Geometry: final body of the model. Coordinates: model frame, mm. Face numbers are marked on the shaded views. A direction names the side the tool comes from. Give positions to 0.01 mm unless a question says otherwise; leave off trailing zeros. Loops run counter-clockwise (first coordinate to the right, second up) from the corner with the lowest first, then second, coordinate; pieces in that order, holes last.
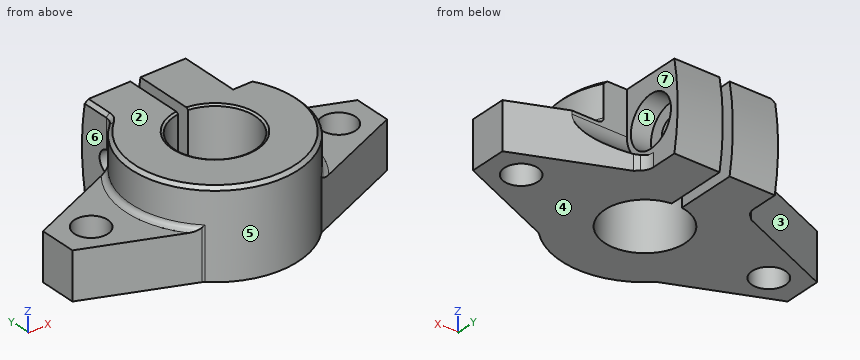
from build123d import *

# Parameters (mm, degrees)
BOSS_EXTRUDE1_DEPTH                                 = 13
CUT_EXTRUDE1_DEPTH                                  = 24.780243901
CUT_EXTRUDE1_DEPTH_BACK                             = 24.780243901
FILLET1_R                                           = 2
BOSS_EXTRUDE2_DEPTH                                 = 7
HOLE_WIZARD_5_0_5_1_D                               = 5
HOLE_WIZARD_5_0_5_1_DEPTH                           = 10
HOLE_WIZARD_5_0_5_1_TIP                             = 1.502151548
CUT_EXTRUDE2_REACH                                  = 39.017
CBORE_FOR_M4_HEX_SOCKET_HEAD_CAP_SCREW3_D           = 3.4
CBORE_FOR_M4_HEX_SOCKET_HEAD_CAP_SCREW3_CBORE_D     = 7.5
CBORE_FOR_M4_HEX_SOCKET_HEAD_CAP_SCREW3_CBORE_DEPTH = 3
CHAMFER2_SIZE                                       = 0.5
FILLET2_R                                           = 0.8
CHAMFER3_SIZE                                       = 0.2
CHAMFER3_SIZE2                                      = 0.346410162


with BuildPart() as part:
    # Sketch1 → Boss-Extrude1 (new body)
    with BuildSketch(Plane.XY):
        with BuildLine():
            Line((0.75, 5.95294045), (0.75, 15.5))
            Line((0.75, 15.5), (7.5, 15.5))
            Line((7.5, 15.5), (7.5, 10))
            ThreePointArc((7.5, 10), (0, -12.5), (-7.5, 10))
            Line((-7.5, 10), (-7.5, 15.5))
            Line((-7.5, 15.5), (-0.75, 15.5))
            Line((-0.75, 15.5), (-0.75, 5.95294045))
            ThreePointArc((-0.75, 5.95294045), (0, -6), (0.75, 5.95294045))
        make_face()
    extrude(amount=BOSS_EXTRUDE1_DEPTH)

    # Sketch2 → Cut-Extrude1 (cut, two sides: drawn at the far end of the back side and taken through both)
    with BuildSketch(Plane(origin=(0, 0, 0), x_dir=(0, 0, -1), z_dir=(1, 0, 0)).offset(-CUT_EXTRUDE1_DEPTH_BACK)):
        with BuildLine():
            Line((69.410215856, 1.772448509), (0, 14.891132578))
            ThreePointArc((0, 14.891132578), (-6.5, 15.5), (-13, 14.891132578))
            Line((-13, 14.891132578), (-82.410215856, 1.772448509))
            Line((-82.410215856, 1.772448509), (-82.410215856, 143.050584636))
            Line((-82.410215856, 143.050584636), (69.410215856, 143.050584636))
            Line((69.410215856, 143.050584636), (69.410215856, 1.772448509))
        make_face()
    extrude(amount=CUT_EXTRUDE1_DEPTH + CUT_EXTRUDE1_DEPTH_BACK, mode=Mode.SUBTRACT)

    # Fillet1
    fillet1_edges = [part.edges().sort_by_distance(p)[0] for p in [
        (7.5, 10, 6.5),
        (-7.5, 10, 6.5),
    ]]
    fillet(fillet1_edges, radius=FILLET1_R)

    # Sketch3 → Boss-Extrude2 (add)
    with BuildSketch(Plane.XY):
        with BuildLine():
            Line((8.803538255, 8.873990883), (23.5, 2.75))
            Line((23.5, 2.75), (23.5, -2.75))
            Line((23.5, -2.75), (8.803538255, -8.873990883))
            ThreePointArc((8.803538255, -8.873990883), (12.5, 0), (8.803538255, 8.873990883))
        make_face()
    extrude(amount=BOSS_EXTRUDE2_DEPTH)

    # Mirror1: part across plane


with BuildPart() as part_1:
    add(part.part)
    add(part.part.mirror(Plane(origin=(0, 0, 0), x_dir=(0, 0, 1), z_dir=(1, 0, 0))))

    # Диаметр отверстия Ø5.0 (5)1
    with Locations(Plane.XY.offset(7)):
        with Locations((18.5, 0), (-18.5, 0)):
            Hole(HOLE_WIZARD_5_0_5_1_D / 2, depth=HOLE_WIZARD_5_0_5_1_DEPTH)
            with Locations((0, 0, -(HOLE_WIZARD_5_0_5_1_DEPTH + HOLE_WIZARD_5_0_5_1_TIP / 2))):  # 118° drill point
                Cone(0, HOLE_WIZARD_5_0_5_1_D / 2, HOLE_WIZARD_5_0_5_1_TIP, mode=Mode.SUBTRACT)

    # Sketch9 → Cut-Extrude2 (cut, up to next)
    with BuildSketch(Plane(origin=(7.5, 0, 0), x_dir=(0, 0, -1), z_dir=(1, 0, 0)), mode=Mode.PRIVATE) as cut_extrude2_sk1:
        with BuildLine():
            Line((-2.023006126, 10.95445115), (-13, 10.95445115))
            Line((-13, 10.95445115), (-13, 6))
            Line((-13, 6), (-6.5, 6))
            ThreePointArc((-6.5, 6), (-3.161210536, 7.482967532), (-2.023006126, 10.95445115))
        make_face()
    cut_extrude2_tool1 = extrude(cut_extrude2_sk1.sketch, amount=CUT_EXTRUDE2_REACH, mode=Mode.PRIVATE) & part_1.part
    add(cut_extrude2_tool1.solids().sort_by_distance((7.5, 8.604622, 7.889878))[0], mode=Mode.SUBTRACT)

    # CBORE for M4 Hex Socket Head Cap Screw3 (through all)
    with Locations(Plane(origin=(7.5, 0, 0), x_dir=(0, 0, -1), z_dir=(1, 0, 0))):
        with Locations((-6.5, 10.5)):
            CounterBoreHole(CBORE_FOR_M4_HEX_SOCKET_HEAD_CAP_SCREW3_D / 2, CBORE_FOR_M4_HEX_SOCKET_HEAD_CAP_SCREW3_CBORE_D / 2, CBORE_FOR_M4_HEX_SOCKET_HEAD_CAP_SCREW3_CBORE_DEPTH)

    # Chamfer2
    chamfer2_edges = [part_1.edges().sort_by_distance(p)[0] for p in [
        (-7.5, 12.922791864, 13),
        (-2.211613172, -12.302795096, 13),
        (-7.680564695, 10.123996352, 13),
    ]]
    chamfer(chamfer2_edges, length=CHAMFER2_SIZE)

    # Fillet2
    fillet2_edges = [part_1.edges().sort_by_distance(p)[0] for p in [
        (12.36996926, -1.798293779, 7),
        (8.803538255, -8.873990883, 3.5),
        (-12.5, 0, 7),
        (-8.803538255, -8.873990883, 3.5),
    ]]
    fillet(fillet2_edges, radius=FILLET2_R)

    # Chamfer3
    chamfer3_edges = [part_1.edges().sort_by_distance(p)[0] for p in [
        (0, -6, 13),
    ]]
    chamfer3_side = [part_1.faces().sort_by_distance(p)[0] for p in [
        (0, -6, 6.5),
    ]]
    chamfer(chamfer3_edges, length=CHAMFER3_SIZE, length2=CHAMFER3_SIZE2, reference=chamfer3_side[0])


solid = part_1.part
Item 1: Ray query, probe 1 along X at (y, z) = (13.75, 10); probe 2 along X at (y, z) = (11.75, 8.5); probe 3 along Y at (x, z) = (-18.5, 4.75). Return the intervals inside material, ascending.
Values follow:
probe 1: x = -7.5 to -0.75, 0.75 to 7.5
probe 2: x = -7.5 to -0.75, 0.75 to 4.5
probe 3: y = -4.83 to -2.5, 2.5 to 4.83
Item 2: Section query C-C on x = 5. Give the number of separate pieces and of enclosed holes in the cut face, plus the area to 3 significant figures.
Values follow:
separate pieces: 2
enclosed holes: 1
area: 217 mm2
Item 3: Set-up query: the marked faces 4, 5, 6 and 7. Return all of +Z, -Z, +X, -X, +Y, -Y with unobstructed straight access to the full face (end or side cutting, diameter ignored); none if empty.
Values follow:
face 4: -Z, +X, -X, +Y, -Y
face 5: +Z
face 6: +Z, -Z, -X, +Y
face 7: +Z, +X, +Y
Item 4: Section query B-B on z = 4. Return loops of the section in (x, y).
Values follow:
outline: (-23.5, -2.75) - (-8.95, -8.81) arc R0.8 cw to (-8.7, -8.98) arc R12.5 ccw to (8.7, -8.98) arc R0.8 cw to (8.95, -8.81) - (23.5, -2.75) - (23.5, 2.75) - (13.88, 6.76) - (7.5, 6.76) - (7.5, 7.7) - (4.5, 7.7) - (4.5, 13.3) - (7.5, 13.3) - (7.5, 15.41) - (0.75, 15.41) - (0.75, 5.95) arc R6 cw (long way) to (-0.75, 5.95) - (-0.75, 15.41) - (-7.5, 15.41) - (-7.5, 10.95) arc R2 cw to (-8.19, 9.44) arc R12.5 ccw to (-8.8, 8.87) - (-23.5, 2.75) - close; hole circle Ø5 at (-18.5, 0); hole circle Ø5 at (18.5, 0)
Item 5: Draft query along Y for the marked faces 1, 2 and 3. Return one class per face: +Y half, -Y half, draft (parallel to the pull), parting line (faces both ways), or undercut.
Values follow:
face 1: undercut
face 2: draft
face 3: +Y half
Item 6: Section query A-A on x = 18.5. Return loops of the section in (y, z).
Values follow:
outline: (-4.83, 0) - (-2.5, 0) - (-2.5, 7) - (-4.83, 7) - close; (2.5, 0) - (4.83, 0) - (4.83, 7) - (2.5, 7) - close
Item 7: Pin query (flat end, axial travel): pin 1 (8 mm diameter, centred on x = -18.5, y = 0, fed in from +Z); pin 2 (2 mm diameter, centred on y = 1, z = 10.5, fed in from -X); pin 3 (1.5 mm diameter, centred on x = -2, z = 3, fed in from +Y); pin 4 (8 mm diameter, centred on x = -1.5, y = -4.5, fed in from -Z). Return the tip coordinate at first contact, or that it passes through.
Values follow:
pin 1: stops at z = 7
pin 2: stops at x = -12.5
pin 3: stops at y = 15.39
pin 4: stops at z = 0
Item 8: Section query D-D on x = 0. Return loops of the section in (y, z), plus the area to 3 significant figures.
Values follow:
outline: (-12.5, 0) - (-6, 0) - (-6, 12.8) - (-6.35, 13) - (-12, 13) - (-12.5, 12.5) - close
area: 84.3 mm2
